Design review of the part built by this model. Coordinates are the model's own, in mm. A direction names the side the tool comes from. Give positions to 0.01 mm unless a question says otherwise; leave off trailing zeros. Loops run counter-clockwise (first coordinate to the right, second up) from the corner with the lowest first, then second, coordinate; pieces in that order, holes last.
from build123d import *

# Parameters (mm, degrees)
BOSS_EXTRUDE1_DEPTH = 4.7625
BOSS_EXTRUDE2_START = -4.7625
BOSS_EXTRUDE2_DEPTH = 4.7625


with BuildPart() as part:
    # Sketch1 → Boss-Extrude1 (new body)
    with BuildSketch(Plane.XY):
        with BuildLine():
            Line((-9.507346898, -10.258391726), (-8.908113007, -12.661787593))
            ThreePointArc((-8.908113007, -12.661787593), (-8.303157018, -13.881491249), (-7.2429575, -14.735672577))
            ThreePointArc((-7.2429575, -14.735672577), (-7.10920631, -14.767138372), (-6.975455121, -14.735672577))
            ThreePointArc((-6.975455121, -14.735672577), (-5.915255603, -13.881491249), (-5.310299614, -12.661787593))
            Line((-5.310299614, -12.661787593), (-4.711065722, -10.258391726))
            ThreePointArc((-4.711065722, -10.258391726), (-4.647570891, -10.043856855), (-4.565714834, -9.835634882))
            ThreePointArc((-4.565714834, -9.835634882), (-3.49859631, -8.649390472), (-1.937719254, -8.318360926))
            ThreePointArc((-1.937719254, -8.318360926), (-1.716465707, -8.351582488), (-1.498925643, -8.403861787))
            Line((-1.498925643, -8.403861787), (0.882093179, -9.086607947))
            ThreePointArc((0.882093179, -9.086607947), (2.240865525, -9.172552521), (3.510708013, -8.681483469))
            ThreePointArc((3.510708013, -8.681483469), (3.604833786, -8.581384439), (3.644459203, -8.449819613))
            ThreePointArc((3.644459203, -8.449819613), (3.434816232, -7.104569234), (2.680999875, -5.970810151))
            Line((2.680999875, -5.970810151), (0.899214945, -4.250160445))
            ThreePointArc((0.899214945, -4.250160445), (0.745169712, -4.087904873), (0.605772222, -3.912904461))
            ThreePointArc((0.605772222, -3.912904461), (0.11201369, -2.395630505), (0.605772222, -0.878356549))
            ThreePointArc((0.605772222, -0.878356549), (0.745169712, -0.703356138), (0.899214945, -0.541100566))
            Line((0.899214945, -0.541100566), (2.680999444, 1.179548724))
            ThreePointArc((2.680999444, 1.179548724), (3.434816124, 2.313307944), (3.644459203, 3.658558603))
            ThreePointArc((3.644459203, 3.658558603), (3.604833786, 3.790123428), (3.510708013, 3.890222459))
            ThreePointArc((3.510708013, 3.890222459), (2.240865525, 4.38129151), (0.882093179, 4.295346937))
            Line((0.882093179, 4.295346937), (-1.498925643, 3.612600776))
            ThreePointArc((-1.498925643, 3.612600776), (-1.716465707, 3.560321477), (-1.937719254, 3.527099916))
            ThreePointArc((-1.937719254, 3.527099916), (-3.49859631, 3.858129461), (-4.565714834, 5.044373871))
            ThreePointArc((-4.565714834, 5.044373871), (-4.647570891, 5.252595845), (-4.711065722, 5.467130715))
            Line((-4.711065722, 5.467130715), (-5.310299614, 7.870526582))
            ThreePointArc((-5.310299614, 7.870526582), (-5.915255603, 9.090230239), (-6.975455121, 9.944411567))
            ThreePointArc((-6.975455121, 9.944411567), (-7.10920631, 9.975877362), (-7.2429575, 9.944411567))
            ThreePointArc((-7.2429575, 9.944411567), (-8.303157018, 9.090230239), (-8.908113007, 7.870526582))
            Line((-8.908113007, 7.870526582), (-9.507346898, 5.467130715))
            ThreePointArc((-9.507346898, 5.467130715), (-9.570841729, 5.252595845), (-9.652697786, 5.044373871))
            ThreePointArc((-9.652697786, 5.044373871), (-10.71981631, 3.858129461), (-12.280693367, 3.527099916))
            ThreePointArc((-12.280693367, 3.527099916), (-12.501946914, 3.560321477), (-12.719486977, 3.612600776))
            Line((-12.719486977, 3.612600776), (-15.100505799, 4.295346937))
            ThreePointArc((-15.100505799, 4.295346937), (-16.459278145, 4.38129151), (-17.729120634, 3.890222459))
            ThreePointArc((-17.729120634, 3.890222459), (-17.823246406, 3.790123428), (-17.862871823, 3.658558603))
            ThreePointArc((-17.862871823, 3.658558603), (-17.653228853, 2.313308223), (-16.899412496, 1.17954914))
            Line((-16.899412496, 1.17954914), (-15.117627565, -0.541100566))
            ThreePointArc((-15.117627565, -0.541100566), (-14.963582333, -0.703356138), (-14.824184843, -0.878356549))
            ThreePointArc((-14.824184843, -0.878356549), (-14.33042631, -2.395630505), (-14.824184843, -3.912904461))
            ThreePointArc((-14.824184843, -3.912904461), (-14.963582333, -4.087904873), (-15.117627565, -4.250160445))
            Line((-15.117627565, -4.250160445), (-16.899412065, -5.970809735))
            ThreePointArc((-16.899412065, -5.970809735), (-17.653228744, -7.104568955), (-17.862871823, -8.449819613))
            ThreePointArc((-17.862871823, -8.449819613), (-17.823246406, -8.581384439), (-17.729120634, -8.681483469))
            ThreePointArc((-17.729120634, -8.681483469), (-16.459278145, -9.172552521), (-15.100505799, -9.086607947))
            Line((-15.100505799, -9.086607947), (-12.719486977, -8.403861787))
            ThreePointArc((-12.719486977, -8.403861787), (-12.501946914, -8.351582488), (-12.280693367, -8.318360926))
            ThreePointArc((-12.280693367, -8.318360926), (-10.71981631, -8.649390472), (-9.652697786, -9.835634882))
            ThreePointArc((-9.652697786, -9.835634882), (-9.570841729, -10.043856855), (-9.507346898, -10.258391726))
        make_face()
        with BuildLine():
            Line((-5.795813757, -3.870630505), (-8.422598864, -3.870630505))
            ThreePointArc((-8.422598864, -3.870630505), (-7.10920631, -0.420630505), (-5.795813757, -3.870630505))
        make_face(mode=Mode.SUBTRACT)
    extrude(amount=BOSS_EXTRUDE1_DEPTH)

    # Sketch4 → Boss-Extrude2 (add)
    with BuildSketch(Plane.XY.offset(4.7625).offset(BOSS_EXTRUDE2_START)):
        with BuildLine():
            Line((-8.422598864, -3.870630505), (-5.795813757, -3.870630505))
            ThreePointArc((-5.795813757, -3.870630505), (-7.10920631, -0.420630505), (-8.422598864, -3.870630505))
        make_face()
        with BuildLine():
            Line((-8.373326558, -3.743630505), (-5.845086063, -3.743630505))
            ThreePointArc((-5.845086063, -3.743630505), (-7.10920631, -0.547630505), (-8.373326558, -3.743630505))
        make_face(mode=Mode.SUBTRACT)
    extrude(amount=BOSS_EXTRUDE2_DEPTH)


solid = part.part
Q1. Insertion check: pin 1 (2 mm diameter, centred on y = -9.5, z = 2.5, fed in from -X); pin 2 (1.5 mm diameter, centred on y = 0, z = 2, fed in from -X). Each pin has a flat end and moves straight along its axis. Give the tip position at first contact, or say it passes through.
Results:
pin 1: stops at x = -17.86
pin 2: stops at x = -16.45
Q2. Wall thickness on line 1 (Y direction, x = 1, z = 3.25); line 2 (Y direction, x = -6, z = 3.45); line 3 (Y direction, x = -14.25, z = 2.45): over which ranges is each line inside the solid? List them lowest first.
Results:
line 1: y = -9.12 to -4.35, -0.44 to 4.33
line 2: y = -13.98 to -3.74, -0.92 to 9.19
line 3: y = -8.84 to 4.05
Q3. Take a section at B-B (x = -7.75). Give the boundary of the cut face in (y, z).
Results:
outline: (-14.42, 0) - (-3.74, 0) - (-3.74, 4.76) - (-14.42, 4.76) - close; (-0.66, 0) - (9.63, 0) - (9.63, 4.76) - (-0.66, 4.76) - close
Q4. Tool access review of faces 1 (the face through (-7, -3.744, 2)), 2 (the face through (-13.89, 3.95, 2.35)), 3 (the face through (-0.33, -8.74, 2.35)): name each direction out of +Z, -Z, +X, -X, +Y, -Y from which nothing blocks a thin tool from reaching the whole face with its end or side.
Results:
face 1: +Z, -Z
face 2: +Z, -Z, +Y
face 3: +Z, -Z, -Y
Q5. Take a section at C-C (x = -2.5). Give the boundary of the cut face in (y, z), plus the area to 3 significant figures.
Results:
outline: (-8.32, 0) - (3.53, 0) - (3.53, 4.76) - (-8.32, 4.76) - close
area: 56.4 mm2
Q6. Take a section at D-D (y = -11.5). Give the boundary of the cut face in (x, z), plus the area to 3 significant figures.
Results:
outline: (-9.2, 0) - (-5.02, 0) - (-5.02, 4.76) - (-9.2, 4.76) - close
area: 19.9 mm2
Q7. Draft analysis for pull direction X (two halves, no side actions). For faces 4 (the face through (-7.05, -0.55, 2.35)), 5 (the face through (1.8, -5.12, 2.35)), 6 (the face through (-17.66, 2.33, 2.35)), state which applies: pulls with the +X half, pulls with the -X half, needs draft (parallel to the pull), parting line crosses it, or undercut.
Results:
face 4: undercut
face 5: pulls with the +X half
face 6: pulls with the -X half
Q8. Take a section at A-A (x = -16.5). Give the boundary of the cut face in (y, z), plus the area to 3 significant figures.
Results:
outline: (-9.17, 0) - (-5.59, 0) - (-5.59, 4.76) - (-9.17, 4.76) - close; (0.79, 0) - (4.37, 0) - (4.37, 4.76) - (0.79, 4.76) - close
area: 34.1 mm2
